The listing builds one solid part. Answer for the finished solid, in the listing's coordinates (mm). A direction names the side the tool comes from. Coordinates: 2 decimals unless noted, no trailing zeros. Write each loop counter-clockwise with the first axis right and the second up, starting at its lowest first coordinate (ties: lowest second). Pieces come first, ordered by that corner, then holes.
(1) The part is cut by section A-A on x = -52.5. Determine the outline of the cut face in (y, z), plus the area to 4 significant figures.
(2) The part is cut by section C-C on z = -45.5. Determine the outline of the cut face in (x, y), plus the area to 3 significant figures.
(3) The part is cut by section D-D on z = -52.5. Determine the outline of the cut face in (x, y).
(4) The part is cut by section B-B on y = 0.4. Determine the outline of the cut face in (x, z), plus the area to 3 significant figures.
(5) Which of the six approach directions +Z, -Z, +X, -X, +Y, -Y give full straight-line access (tool end or side, diameter ignored) to faces 4 (the flat face through (-55.895, -1, -68)), 5 (the flat face through (-45.895, -1, -68)), 6 (the flat face through (-50, 1.2, -45)), 7 (the cylindrical face through (-39.183, 0.608, -44.042)), 8 (the flat face through (-51, 2, -64.229))?
(6) Straight lines are drawn through the part: line 1 (Y direction, x = -56, z = -55.25); line 2 (Z direction, x = -52.75, y = 1.4); line 3 (Y direction, x = -60.75, z = -45.25). For each, find the intervals that lie inside material, in ascending order.
(7) Given P1, Ø2.5, axis at x = -51.5, z = -44.5, coming from the +Y side; P2, Ø1.2, axis at x = -51, y = -1.5, coming from the +Z side; P3, Ø1.2, axis at y = -1.5, z = -68, coming from the +X side, each flat-ended and moving along its own axis, determine where each tip first touches the part or whether it passes through.
(8) For a pull along X with two mould halves and no side action, classify faces 1 (the flat face through (-37.645, 1, -56)), 2 (the cylindrical face through (-61.183, 0.608, -66.042)), 3 (the flat face through (-51, -1, -66.429)) as +X half, -X half, draft (parallel to the pull), parting line (faces both ways), or undercut.
Autodesk Inventor part; units mm, degrees
ref_plane "YZ Plane" through (0, 0, 0) normal (1, 0, 0) x (0, 1, 0)
ref_plane "XZ Plane" through (0, 0, 0) normal (0, 1, 0) x (-1, 0, 0)
ref_plane "XY Plane" through (0, 0, 0) normal (0, 0, 1) x (1, 0, 0)
sketch "Sketch1" plane through (0, 0, 0) normal (0, 1, 0) x (-1, 0, 0)
  line L0 (63.6448, -68.929) -> (37.6448, -68.929)
  line L1 (37.6448, -68.929) -> (37.6448, -42.929)
  line L2 (37.6448, -42.929) -> (63.6448, -42.929)
  line L3 (63.6448, -42.929) -> (63.6448, -68.929)
  point P0 (0, 0)
  dimension "d0" = 26
  dimension "d1" = 26
extrude "Extrusion1" add sketch "Sketch1" along normal blind 1.2
sketch "Sketch2" plane through (0, 1.2, 0) normal (0, 1, 0) x (1, 0, 0)
  line L0 (-63.6448, 68.929) -> (-63.6448, 42.929)
  line L1 (-37.6448, 42.929) -> (-37.6448, 68.929)
  line L2 (-63.6448, 64.229) -> (-37.6448, 64.229)
  line L3 (-37.6448, 64.229) -> (-37.6448, 47.629)
  line L4 (-37.6448, 47.629) -> (-63.6448, 47.629)
  line L5 (-63.6448, 47.629) -> (-63.6448, 64.229)
  line L6 (-37.6448, 68.929) -> (-63.6448, 68.929)
  point P0 (0, 0)
  point P1 (-63.6448, 47.629)
  dimension "d4" = 4.7
  dimension "d5" = 16.6
extrude "Extrusion2" add sketch "Sketch2" along normal blind 2 contours L2 L1 L4 L0
sketch "Sketch3" plane through (0, 1.2, 0) normal (0, 1, 0) x (1, 0, 0)
  circle A0 centre (-61.6448, 66.929) radius 1
  circle A1 centre (-39.6448, 66.929) radius 1
  circle A2 centre (-39.6448, 44.929) radius 1
  circle A3 centre (-61.8448, 44.929) radius 1
  line L0 (-63.6448, 68.929) -> (-63.6448, 64.229)
  line L1 (-37.6448, 68.929) -> (-63.6448, 68.929)
  line L2 (-37.6448, 64.229) -> (-37.6448, 68.929)
  line L3 (-37.6448, 42.929) -> (-37.6448, 47.629)
  line L4 (-63.6448, 42.929) -> (-37.6448, 42.929)
  line L5 (-63.6448, 47.629) -> (-63.6448, 42.929)
  point P0 (0, 0)
  point P1 (-63.6448, 45.279)
  dimension "d8" = 2
  dimension "d9" = 2
  dimension "d10" = 2
  dimension "d11" = 2
  dimension "d12" = 2
  dimension "d13" = 2
  dimension "d14" = 2
  dimension "d15" = 2
  dimension "d16" = 2
  dimension "d17" = 2
  dimension "d18" = 2
  dimension "d19" = 1.8
extrude "Extrusion3" cut sketch "Sketch3" against normal through all
sketch "Sketch4" plane through (0, 0, 0) normal (0, -1, 0) x (1, 0, 0)
  line L0 (-45.8948, -68.929) -> (-55.8948, -68.929)
  line L1 (-55.8948, -68.929) -> (-55.8948, -66.429)
  line L2 (-55.8948, -66.429) -> (-45.8948, -66.429)
  line L3 (-45.8948, -66.429) -> (-45.8948, -68.929)
  line L4 (-37.6448, -68.929) -> (-63.6448, -68.929)
  line L5 (-37.6448, -42.929) -> (-37.6448, -68.929)
  point P0 (0, 0)
  dimension "d22" = 10
  dimension "d23" = 2.5
  dimension "d24" = 0
  dimension "d25" = 8.25
extrude "Extrusion4" add sketch "Sketch4" along normal blind 2.5
equation "\"d14\" = d13"
equation "\"d15\" = d14"
equation "\"d16\" = d14"
equation "\"d17\" = d15"
equation "\"d18\" = d12"
properties part number "ssd1360"
Model answer:
1. outline: (-2.5, -68.93) - (1.2, -68.93) - (1.2, -64.23) - (3.2, -64.23) - (3.2, -47.63) - (1.2, -47.63) - (1.2, -42.93) - (0, -42.93) - (0, -66.43) - (-2.5, -66.43) - close
1. area: 70.65 mm2
2. outline: (-63.64, 0) - (-62.67, 0) - (-62.67, 1.2) - (-63.64, 1.2) - close; (-61.02, 0) - (-40.47, 0) - (-40.47, 1.2) - (-61.02, 1.2) - close; (-38.82, 0) - (-37.64, 0) - (-37.64, 1.2) - (-38.82, 1.2) - close
2. area: 27.3 mm2
3. outline: (-63.64, 0) - (-37.64, 0) - (-37.64, 3.2) - (-63.64, 3.2) - close
4. outline: (-63.64, -68.93) - (-37.64, -68.93) - (-37.64, -42.93) - (-63.64, -42.93) - close; hole circle Ø2 at (-61.84, -44.93); hole circle Ø2 at (-61.64, -66.93); hole circle Ø2 at (-39.64, -66.93); hole circle Ø2 at (-39.64, -44.93)
4. area: 663 mm2
5. face 4: +Z, -Z, -X, -Y
5. face 5: +Z, -Z, +X, -Y
5. face 6: +Z, +X, -X, +Y
5. face 7: +Y, -Y
5. face 8: -Z, +X, -X, +Y
6. line 1: y = 0 to 3.2
6. line 2: z = -64.23 to -47.63
6. line 3: y = 0 to 1.2
7. P1: stops at y = 1.2
7. P2: stops at z = -66.43
7. P3: stops at x = -45.89
8. face 1: +X half
8. face 2: undercut
8. face 3: draft
